Can you work these out from the model? Positions are in its coordinate system, mm. A direction names the side the tool comes from. Coordinates: 2 decimals unless noted, no trailing zeros. Order: outer loops, then holes, each group sorted by start corner. A loop starts at its lowest first (then second) coordinate and runs counter-clockwise, first axis right, second up. Notation, with made-up numbers: (-36, 3.25) -> (20, 3.25) arc R12 cw to (20, 11.25) -> close; hole circle Ø4 at (-11.75, 0). An arc over 180 degrees is marked (long way). Answer in a Markdown table with one row per item. Add a question column.
1. Imagine slicing it at D-D on z = 55. Write out the boundary of the cut face in (x, y), plus the area to 3 significant figures.
2. If I drill on line 1 along Y through (x, z) = (0, 4); line 2 along X through (y, z) = (27.5, 4.25); line 3 along Z through (x, y) = (-2.5, 23), over which ranges is the centre line in solid material (lowest first)? Write a range as [from, to].
3. On a 3-axis mill with a long thin cutter (end or side, diameter ignored), from which of +Z, -Z, +X, -X, +Y, -Y can I reach the whole of each face in a straight line? I mean faces 1 (the face through (-10, 27, 2)), 2 (the face through (18, 52, 0)), 3 (the face through (24, 53, 50)). Say none if no direction works.
4. Imagine slicing it at A-A on y = 27.5. Write out the boundary of the cut face in (x, z).
5. Imagine slicing it at B-B on x = 0. Write out the boundary of the cut face in (y, z).
6. Will these pins go through, and if not, where does the flat tip stop? pin 1 (16.5 mm diameter, centred on x = 20, y = 55.5, fed in from -Z); pin 2 (1 mm diameter, centred on x = 28.5, z = 18.5, fed in from -Y); pin 3 (14.5 mm diameter, centred on y = 27.5, z = 2.5, fed in from +X).
Autodesk Inventor part; units mm, degrees
ref_plane "YZ Plane" through (0, 0, 0) normal (1, 0, 0) x (0, 1, 0)
ref_plane "XZ Plane" through (0, 0, 0) normal (0, 1, 0) x (-1, 0, 0)
ref_plane "XY Plane" through (0, 0, 0) normal (0, 0, 1) x (1, 0, 0)
sketch "Sketch9" plane through (0, 0, 0) normal (0, 0, 1) x (1, 0, 0)
  line L0 (0, 0) -> (0, 55) construction
  circle A0 centre (0, 55) radius 1.5
  circle A1 centre (0, 0) radius 1.5
  circle A2 centre (0, 27.5) radius 1.5
  line L1 (-10, 60) -> (10, 60)
  line L2 (10, 60) -> (10, -5)
  line L3 (10, -5) -> (-10, -5)
  line L4 (-10, -5) -> (-10, 60)
  point P0 (-10, 27.5)
  point P1 (0, 60)
  dimension "d35" = 55
  dimension "d36" = 3
  dimension "d37" = 3
  dimension "d38" = 3
  dimension "d39" = 5
  dimension "d40" = 10
extrude "Extrusion9" add sketch "Sketch9" along normal blind 10
sketch "Sketch11" plane through (10, -5, 0) normal (1, 0, 0) x (0, 0, -1)
  line L0 (0, 65) -> (-10, 65)
  line L1 (0, 65) -> (-75, 65)
  line L2 (-75, 65) -> (-75, 50)
  line L3 (-75, 50) -> (0, 50)
  line L4 (0, 50) -> (0, 65)
  point P0 (0, 5)
  dimension "d43" = 15
  dimension "d44" = 75
extrude "Extrusion10" add sketch "Sketch11" along normal blind 35
sketch "Sketch12" plane through (-10, 60, 10) normal (0, 1, 0) x (1, 0, 0)
  line L0 (20, -65) -> (20, 0)
  line L1 (20, -65) -> (34, -65)
  line L2 (34, -65) -> (34, 0)
  line L3 (34, 0) -> (20, 0)
  line L4 (20, 0) -> (20, -65)
  point P0 (10, 10)
  dimension "d47" = 14
extrude "Extrusion11" cut sketch "Sketch12" against normal through all
chamfer "Chamfer6" distance 14 angle 45 1 edges at (24, 52.5, 10)
sketch "Sketch14" plane through (10, 45, 0) normal (0, -1, 0) x (1, 0, 0)
  line L0 (0, 10) -> (14, 24)
  line L1 (15.4558, 0) -> (35, 19.5442)
  line L2 (35, 75) -> (35, 0)
  line L3 (0, 0) -> (35, 0)
  line L4 (15.4558, 0) -> (35, 0)
  line L5 (35, 19.5442) -> (35, 0)
  point P0 (-10, 0)
  dimension "d73" = 18
extrude "Extrusion13" cut sketch "Sketch14" against normal through all
sketch "Sketch15" plane through (0, 0, 0) normal (0, 0, -1) x (-1, 0, 0)
  line L0 (-25.4558, 60) -> (-25.4558, 45)
  line L1 (-10, 45) -> (-25.4558, 45)
  line L2 (-10, 45) -> (-10, -5)
  line L3 (-10, -5) -> (10, -5)
  line L4 (10, -5) -> (10, 60)
  line L5 (10, 60) -> (-25.4558, 60)
  circle A0 centre (0, 55) radius 1.5
  circle A1 centre (0, 0) radius 1.5
  circle A2 centre (0, 27.5) radius 1.5
  line L6 (-10, -5) -> (10, -5)
  line L7 (10, 60) -> (-10, 60)
  line L8 (-10, -5) -> (-10, 60)
  line L9 (-10, 60) -> (10, 60)
extrude "Extrusion14" add sketch "Sketch15" along normal blind 3 contours L5 L4 L3 L2 L8
chamfer "Chamfer8" distance 3 angle 45 1 edges at (-10, 27.5, 10)
sketch "Sketch17" plane through (-10, -5, -3) normal (0, -1, 0) x (1, 0, 0)
  line L0 (20, 3) -> (20, 13)
  line L1 (20, 3) -> (35.4558, 3)
  line L2 (20, 3) -> (35.4558, 3)
  line L3 (35.4558, 3) -> (37.5981, 1.5)
  line L4 (37.5981, 1.5) -> (49, 1.5)
  line L5 (49, 3.5) -> (38.2287, 3.5)
  line L6 (38.2287, 3.5) -> (36.0864, 5)
  line L7 (36.0864, 5) -> (20, 5)
  line L8 (20, 3) -> (20, 5)
  line L9 (49, 3.5) -> (49, 1.5)
  line L10 (55, 78) -> (55, 22.5442)
  point P0 (10, 3)
  dimension "d83" = 145
  dimension "d84" = 2
  dimension "d87" = 1.5
  dimension "d88" = 6
extrude "Extrusion16" add sketch "Sketch17" against normal blind 65
sketch "Sketch18" plane through (24, 45, 75) normal (0, -1, 0) x (1, 0, 0)
  line L0 (-34, -68) -> (-31, -65)
  line L1 (-34, -68) -> (-34, -78)
  line L2 (-14, -78) -> (-34, -78)
  line L3 (-14, -75) -> (-14, -78)
  line L4 (-14, -75) -> (1.4558, -75)
  line L5 (1.4558, -75) -> (3.5981, -76.5)
  line L6 (3.5981, -76.5) -> (15, -76.5)
  line L7 (15, -76.5) -> (15, -74.5)
  line L8 (15, -74.5) -> (4.2287, -74.5)
  line L9 (4.2287, -74.5) -> (2.0864, -73)
  line L10 (2.0864, -73) -> (-14, -73)
  line L11 (-14, -65) -> (-14, -73)
  line L12 (-31, -65) -> (-14, -65)
  line L13 (2.8919, -73.564) -> (4.2287, -74.5)
  line L14 (2.8919, -73.564) -> (1.4558, -75)
  point P0 (-24, -75)
extrude "Extrusion17" cut sketch "Sketch18" against normal through all contours L14 L9 L8 L7 L6 L5
sketch "Sketch19" plane through (-10, -5, -3) normal (0, -1, 0) x (1, 0, 0)
  line L0 (0, 10) -> (3, 13)
  line L1 (0, 10) -> (0, 0)
  line L2 (20, 0) -> (0, 0)
  line L3 (20, 3) -> (20, 0)
  line L4 (20, 3) -> (35.4558, 3)
  line L5 (35.4558, 3) -> (37.5981, 1.5)
  line L6 (37.5981, 1.5) -> (49, 1.5)
  line L7 (49, 1.5) -> (49, 3.5)
  line L8 (49, 3.5) -> (38.2287, 3.5)
  line L9 (38.2287, 3.5) -> (36.0864, 5)
  line L10 (36.0864, 5) -> (20, 5)
  line L11 (20, 13) -> (20, 5)
  line L12 (3, 13) -> (20, 13)
  line L13 (20, 5) -> (20, 3)
  point P0 (10, 3)
extrude "Extrusion18" cut sketch "Sketch19" against normal blind 50 contours L10 L9 L8 L7 L6 L5 L4 L13
equation "\"Module\" = 2"
equation "\"PressureAngle\" = 20deg"
equation "\"UnitProfileClearance\" = 0.25"
equation "\"UnitRoundRadius\" = 0.35"
equation "\"HeadDiameter\" = 42"
equation "\"RootDiameter\" = 33"
equation "\"BaseDiameter\" = 35.70832"
equation "\"PitchDiameter\" = 38"
equation "\"HelixAngle\" = 0"
equation "\"UnitCorrection\" = 0"
equation "\"UnitAddendumModification\" = 0"
equation "\"CircularPitch\" = 6.283185"
equation "\"UnitBacklashShift\" = 0"
equation "\"TotalToolShift\" = 0"
equation "\"IsInternal\" = 0"
properties part number "GA04" material "ABS Plastic"
Answers follow:
| question | item | result |
|---|---|---|
| 1 | outline | (24, 45) -> (45, 45) -> (45, 60) -> (24, 60) -> close |
| 1 | area | 315 mm² |
| 2 | line 1 | y = [-5, -1.5], [1.5, 26], [29, 53.5], [56.5, 60] |
| 2 | line 2 | x = [-10, -1.5], [1.5, 10] |
| 2 | line 3 | z = [-3, 10] |
| 3 | face 1 | +Z, -Z, -X, +Y, -Y |
| 3 | face 2 | -Z, +X, +Y, -Y |
| 3 | face 3 | +Z, -X, +Y, -Y |
| 4 | outline | (-10, -3) -> (-1.5, -3) -> (-1.5, 10) -> (-7, 10) -> (-10, 7) -> close; (1.5, -3) -> (10, -3) -> (10, 10) -> (1.5, 10) -> close |
| 5 | outline | (-5, -3) -> (-1.5, -3) -> (-1.5, 10) -> (-5, 10) -> close; (1.5, -3) -> (26, -3) -> (26, 10) -> (1.5, 10) -> close; (29, -3) -> (53.5, -3) -> (53.5, 10) -> (29, 10) -> close; (56.5, -3) -> (60, -3) -> (60, 10) -> (56.5, 10) -> close |
| 6 | pin 1 | stops at z = 0 |
| 6 | pin 2 | stops at y = 45 |
| 6 | pin 3 | stops at x = 10 |
